Read the model definition and answer for the solid it produces. Units are mm, in the model's axes. Face numbers are marked on the shaded views. A direction names the side the tool comes from. Give positions to 0.01 mm unless a question says otherwise; leave off trailing zeros. Order: outer loops, then holes, each group sorted by start corner. A loop starts at its lowest first (then second) coordinate and runs counter-clockwise, first axis right, second up. Notation, with made-up numbers: (31.25, 43) - (82.25, 43) arc R13 cw to (82.25, 65) - close; hole circle Ø3 at (69.25, 11.25). An arc over 180 degrees is marked (long way). Write item = value, one per line.
```python
from build123d import *

# Parameters (mm, degrees)
EXTRUDE_1_DEPTH     = 41
SKETCH_2_R          = 6.05
SKETCH_2_R_2        = 1.6
CUT_EXTRUDE_1_DEPTH = 41
SKETCH_3_R          = 1.6
CUT_EXTRUDE_2_DEPTH = 41


with BuildPart() as part:
    # ｽｹｯﾁ1 → ﾎﾞｽ - 押し出し1 (new body)
    with BuildSketch(Plane.XY):
        Polygon((0, 0), (0, 42), (3, 42), (3, 3), (36.6, 3), (36.6, 0), align=None)
    extrude(amount=EXTRUDE_1_DEPTH)

    # ｽｹｯﾁ2 → ｶｯﾄ - 押し出し1 (cut)
    with BuildSketch(Plane.ZY):
        with Locations((20.5, 28.5)):
            Circle(SKETCH_2_R)
        with Locations((28.25, 34.925)):
            Circle(SKETCH_2_R_2)
        with Locations((28.25, 8.075)):
            Circle(SKETCH_2_R_2)
        with Locations((12.75, 8.075)):
            Circle(SKETCH_2_R_2)
        with Locations((12.75, 34.925)):
            Circle(SKETCH_2_R_2)
    extrude(amount=-CUT_EXTRUDE_1_DEPTH, mode=Mode.SUBTRACT)

    # ｽｹｯﾁ3 → ｶｯﾄ - 押し出し2 (cut)
    with BuildSketch(Plane(origin=(0, 0, 0), x_dir=(-1, 0, 0), z_dir=(0, -1, 0))):
        with Locations((-10.6, -37)):
            Circle(SKETCH_3_R)
        with Locations((-10.6, -4)):
            Circle(SKETCH_3_R)
        with Locations((-29, -4)):
            Circle(SKETCH_3_R)
        with Locations((-29, -37)):
            Circle(SKETCH_3_R)
    extrude(amount=-CUT_EXTRUDE_2_DEPTH, mode=Mode.SUBTRACT)


solid = part.part
```
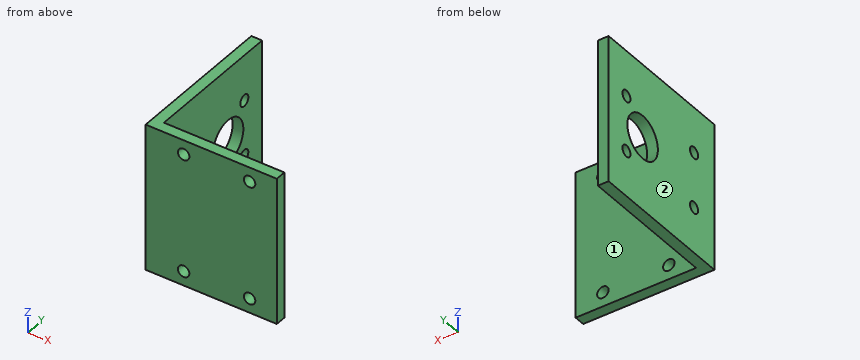
1. Flat-ended cylindrical pins translate along their axes: pin 1 (7.5 mm diameter, centred on y = 28.5, z = 20.5, fed in from -X); pin 2 (8 mm diameter, centred on y = 37.5, z = 21.5, fed in from +X); pin 3 (10 mm diameter, centred on x = 23.5, z = 28.5, fed in from +Y). Find the tip coordinate at first contact, or state that the pin passes through.
Recorded:
pin_1 = through
pin_2 = 3
pin_3 = 3
2. Section A-A (x = 10.6) is taken. Determine the outline of the cut face in (y, z), and give its area (3 significant figures).
Recorded:
outline = (0, 0) - (3, 0) - (3, 2.4) - (0, 2.4) - close; (0, 5.6) - (3, 5.6) - (3, 35.4) - (0, 35.4) - close; (0, 38.6) - (3, 38.6) - (3, 41) - (0, 41) - close
area = 104 mm^2
3. Straight lines are drawn through the part: L1, parallel to Z at x = 29, y = 2; L2, parallel to X at y = 1.65, z = 4; L3, parallel to Y at x = 2.05, z = 12.75 (3 decimals). For each, find the intervals that lie inside material, in ascending order. Write a range as [from, to].
Recorded:
L1 = [0, 2.4], [5.6, 35.4], [38.6, 41]
L2 = [0, 9], [12.2, 27.4], [30.6, 36.6]
L3 = [0, 6.475], [9.675, 33.325], [36.525, 42]
4. Section C-C (y = 30) is taken. Determine the outline of the cut face in (x, z), and give its area (3 significant figures).
Recorded:
outline = (0, 0) - (3, 0) - (3, 14.64) - (0, 14.64) - close; (0, 26.36) - (3, 26.36) - (3, 41) - (0, 41) - close
area = 87.8 mm^2
5. For the marked faces 1 and 2, determine the directions among +Z, -Z, +X, -X, +Y, -Y from which every point of the face is accessible in a straight line to the end or side of a thin tool.
Recorded:
face_1 = +Z, -Z, +X, +Y
face_2 = +Z, -Z, -X, +Y, -Y
6. Section B-B (z = 4) is taken. Determine the outline of the cut face in (x, y).
Recorded:
outline = (0, 0) - (9, 0) - (9, 3) - (3, 3) - (3, 42) - (0, 42) - close; (12.2, 0) - (27.4, 0) - (27.4, 3) - (12.2, 3) - close; (30.6, 0) - (36.6, 0) - (36.6, 3) - (30.6, 3) - close
7. Section D-D (z = 25.5) is taken. Determine the outline of the cut face in (x, y), and give its area (3 significant figures).
Recorded:
outline = (0, 0) - (36.6, 0) - (36.6, 3) - (3, 3) - (3, 25.09) - (0, 25.09) - close; (0, 31.91) - (3, 31.91) - (3, 42) - (0, 42) - close
area = 206 mm^2
